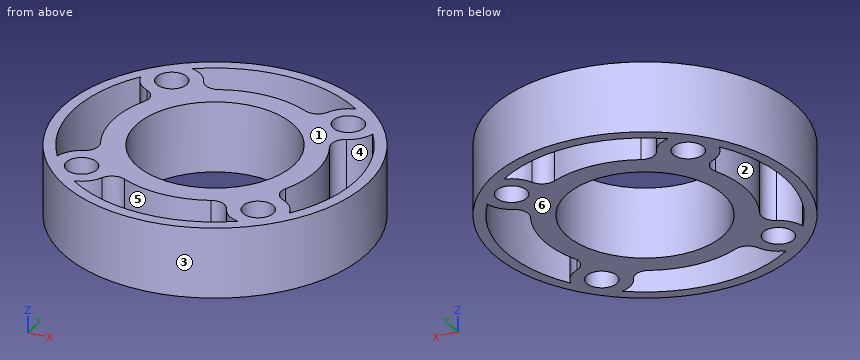
```python
from build123d import *

# Parameters (mm, degrees)
F0_R            = 21.43125
F0_R_2          = 2.15265
F0_R_3          = 11.1125
F1_DEPTH        = 9.9568
F3_DEPTH        = 9.9568
F3_COPIES_COUNT = 4
F4_R            = 1.984375


# Not quite as in the source:
# - a pattern or mirror of a feature is missing from the dataset's text; its kind, count and spacing are read off the source's solid


with BuildPart() as f1:
    # F0 (on Top) → F1 (new body)
    with BuildSketch(Plane.XY):
        Circle(F0_R)
        with Locations((-12.3478521665, -12.3478521665)):
            Circle(F0_R_2, mode=Mode.SUBTRACT)
        with Locations((12.3478521665, -12.3478521665)):
            Circle(F0_R_2, mode=Mode.SUBTRACT)
        with Locations((-12.3478521665, 12.3478521665)):
            Circle(F0_R_2, mode=Mode.SUBTRACT)
        Circle(F0_R_3, mode=Mode.SUBTRACT)
        with Locations((12.3478521665, 12.3478521665)):
            Circle(F0_R_2, mode=Mode.SUBTRACT)
    extrude(amount=F1_DEPTH)

    # F2 (on face) → F3 (cut, through all)
    with BuildSketch(Plane.XY.offset(9.9568)):
        with BuildLine():
            ThreePointArc((8.4692641257, 11.5067033254), (8.9929440308, 14.4681276118), (11.4430257563, 16.212081162))
            ThreePointArc((11.4430257563, 16.212081162), (0, 19.84375), (-11.4430257563, 16.212081162))
            ThreePointArc((-11.4430257563, 16.212081162), (-8.9929440308, 14.4681276118), (-8.4692641257, 11.5067033254))
            ThreePointArc((-8.4692641257, 11.5067033254), (0, 14.2875), (8.4692641257, 11.5067033254))
        make_face()
    f3 = extrude(amount=-F3_DEPTH, mode=Mode.SUBTRACT)

    # F3_copies: F3 ×4 about axis
    f3_copies_axis = Axis((0, 0, 0), (0, 0, 1))
    for i in range(1, F3_COPIES_COUNT):
        add(f3.rotate(f3_copies_axis, i * 360 / F3_COPIES_COUNT), mode=Mode.SUBTRACT)

    # F4
    f4_edges = [f1.edges().sort_by_distance(p)[0] for p in [
        (8.469264, 11.506703, 4.9784),
        (-8.469264, 11.506703, 4.9784),
        (8.469264, -11.506703, 4.9784),
        (-8.469264, -11.506703, 4.9784),
        (11.506703, 8.469264, 4.9784),
        (11.506703, -8.469264, 4.9784),
        (-11.506703, -8.469264, 4.9784),
        (-11.506703, 8.469264, 4.9784),
    ]]
    fillet(f4_edges, radius=F4_R)


solid = f1.part
```
Model file for the job. Use its own axes, mm. Face numbers are marked on the shaded views. A direction names the side the tool comes from. Coordinates: 2 decimals unless noted, no trailing zeros. Write each loop counter-clockwise with the first axis right and the second up, starting at its lowest first coordinate (ties: lowest second). Pieces come first, ordered by that corner, then holes. Notation, with made-up numbers: (-6.75, 52.25) - (2.25, 52.25) arc R29 cw to (2.25, 77.25) - close; hole circle Ø2 at (48.5, -7). An arc over 180 degrees is marked (long way). Use a Markdown table: item, result. Add a question column.
Item 1: Drop flat-ended pins along their axis: pin 1 (2 mm diameter, centred on y = -3.5, z = 8.5, fed in from -X); pin 2 (1 mm diameter, centred on y = -17, z = 4.5, fed in from +X); pin 3 (1.5 mm diameter, centred on x = 17, z = 8.5, fed in from -Y). Give the stop position or say it passes through.
Item 2: Band-saw the part on A-A, the plane y = 0. Write the cut outline in (x, z), and give its area (3 significant figures).
Item 3: 3-axis set-ups, long thin cutter, end or side, ignore diameter. For the marked faces 1 and 2: which of +Z, -Z, +X, -X, +Y, -Y reach the whole face in a straight line?
Item 4: Drill centre lines: line 1 along Y through (x, z) = (-0.5, 5); line 2 along Y through (x, z) = (-10, 2.5); line 3 along X through (y, z) = (-4.5, 1.25). Where is each one in solid material? Low to high.
Item 5: Band-saw the part on D-D, the plane x = 18.5. Write the cut outline in (y, z).
Item 6: Band-saw the part on C-C, the plane y = 18. Write the cut outline in (x, z), and give its area (3 significant figures).
Item 7: Two-plate mould, pull along Y, no slides. Class the marked faces 3, 4, 5 and 6: pulls with the +Y half, pulls with the -Y half, needs draft (parallel to the pull), parting line crosses it, or undercut.
A:
| question | item | result |
|---|---|---|
| 1 | pin 1 | stops at x = -21.28 |
| 1 | pin 2 | stops at x = 13.68 |
| 1 | pin 3 | stops at y = -13.97 |
| 2 | outline | (-21.43, 0) - (-19.84, 0) - (-19.84, 9.96) - (-21.43, 9.96) - close; (-14.29, 0) - (-11.11, 0) - (-11.11, 9.96) - (-14.29, 9.96) - close; (11.11, 0) - (14.29, 0) - (14.29, 9.96) - (11.11, 9.96) - close; (19.84, 0) - (21.43, 0) - (21.43, 9.96) - (19.84, 9.96) - close |
| 2 | area | 94.8 mm² |
| 3 | face 1 | +Z, +X, -X, +Y, -Y |
| 3 | face 2 | +Z, -Z |
| 4 | line 1 | y = -21.43 to -19.84, -14.28 to -11.1, 11.1 to 14.28, 19.84 to 21.43 |
| 4 | line 2 | y = -18.96 to -17.14, -15.55 to -4.85, 4.85 to 15.55, 17.14 to 18.96 |
| 4 | line 3 | x = -20.95 to -19.33, -13.56 to -10.16, 10.16 to 13.56, 19.33 to 20.95 |
| 5 | outline | (-10.82, 0) - (-7.18, 0) - (-7.18, 9.96) - (-10.82, 9.96) - close; (7.18, 0) - (10.82, 0) - (10.82, 9.96) - (7.18, 9.96) - close |
| 6 | outline | (-11.63, 0) - (-8.35, 0) - (-8.35, 9.96) - (-11.63, 9.96) - close; (8.35, 0) - (11.63, 0) - (11.63, 9.96) - (8.35, 9.96) - close |
| 6 | area | 65.3 mm² |
| 7 | face 3 | parting line crosses it |
| 7 | face 4 | undercut |
| 7 | face 5 | undercut |
| 7 | face 6 | needs draft |
